CAD build for the part. Positions are in the model's coordinates, mm. A direction names the side the tool comes from. Round coordinates to 2 decimals unless told otherwise and drop trailing zeros. Loops run counter-clockwise (first coordinate to the right, second up) from the corner with the lowest first, then second, coordinate; pieces in that order, holes last.
from build123d import *

# Parameters (mm, degrees)
F0_W      = 153.5
F0_H      = 82
F1_DEPTH  = 2
F2_R      = 7
F2_R_2    = 1.75
F3_DEPTH  = 2.001
F4_SIZE   = 1.99999
F5_R      = 2
F6_DEPTH  = 33
F7_W      = 153.5
F7_H      = 82
F7_W_2    = 149.5
F7_H_2    = 78
F8_DEPTH  = 31
F10_DEPTH = 82.001
F12_DEPTH = 153.501
F13_W     = 56
F13_H     = 56
F13_W_2   = 52
F13_H_2   = 52
F14_DEPTH = 30
F16_DEPTH = 82.001
F17_R     = 5


# Not quite as in the source:
# - a fillet or chamfer is up to 0.001 mm smaller than in the source, because OpenCascade refuses the exact size


with BuildPart() as f1:
    # F0 (on Top) → F1 (new body)
    with BuildSketch(Plane.XY):
        Rectangle(F0_W, F0_H)
    extrude(amount=F1_DEPTH)

    # F2 (on face) → F3 (cut, through all)
    with BuildSketch(Plane.XY.offset(2)):
        with Locations((-48.75, -13)):
            Circle(F2_R)
        with Locations((-68.75, -13)):
            Circle(F2_R_2)
        with Locations((-28.75, -13)):
            Circle(F2_R_2)
    extrude(amount=-F3_DEPTH, mode=Mode.SUBTRACT)

    # F4 (size 2 in the source; OpenCascade refuses exactly that, so slightly less here)
    f4_edges = [f1.edges().sort_by_distance(p)[0] for p in [
        (-70.5, -13, 0),
        (-30.5, -13, 0),
    ]]
    chamfer(f4_edges, length=F4_SIZE)

    # F5 (on face) → F6 (join)
    with BuildSketch(Plane.XY.offset(2)):
        with Locations((-74.75, 39)):
            Circle(F5_R)
        with Locations((74.75, 39)):
            Circle(F5_R)
        with Locations((-74.75, -39)):
            Circle(F5_R)
        with Locations((74.75, -39)):
            Circle(F5_R)
    extrude(amount=F6_DEPTH)

    # F7 (on face) → F8 (join)
    with BuildSketch(Plane.XY.offset(2)):
        Rectangle(F7_W, F7_H)
        Rectangle(F7_W_2, F7_H_2, mode=Mode.SUBTRACT)
    extrude(amount=F8_DEPTH)

    # F9 (on face) → F10 (cut, through all)
    with BuildSketch(Plane.XZ.offset(41)):
        with BuildLine():
            Line((70, 33), (-70, 33))
            ThreePointArc((-70, 33), (0, 5), (70, 33))
        make_face()
    extrude(amount=-F10_DEPTH, mode=Mode.SUBTRACT)

    # F11 (on face) → F12 (cut, through all)
    with BuildSketch(Plane.YZ.offset(76.75)):
        with BuildLine():
            Line((35, 33), (-35, 33))
            ThreePointArc((-35, 33), (0, 5), (35, 33))
        make_face()
    extrude(amount=-F12_DEPTH, mode=Mode.SUBTRACT)

    # F13 (on face) → F14 (join)
    with BuildSketch(Plane.XY.offset(2)):
        with Locations((-48.75, -13)):
            Rectangle(F13_W, F13_H)
        with Locations((-48.75, -13)):
            Rectangle(F13_W_2, F13_H_2, mode=Mode.SUBTRACT)
    extrude(amount=F14_DEPTH)

    # F15 (on face) → F16 (cut, through all)
    with BuildSketch(Plane.XZ.offset(41)):
        Polygon((-20.75, 28), (-20.75, 32), (-44.8423758792, 32), align=None)
    extrude(amount=-F16_DEPTH, mode=Mode.SUBTRACT)

    # F17
    f17_edges = [f1.edges().sort_by_distance(p)[0] for p in [
        (-20.75, -40, 7.143634),
        (-75.75, 15, 8.286419),
    ]]
    fillet(f17_edges, radius=F17_R)


solid = f1.part
Item 1: Mould opens along X. For faces 5 (the cylindrical face through (-75.74, 17.83, 12.85)), 6 (the flat face through (-49, 15, 17)), 7 (the flat face through (76.75, -1, 2)) say: released by +X, released by -X, zero draft, split by the parting line, or undercut.
Verdict:
face 5: zero draft
face 6: undercut
face 7: released by +X
Item 2: Cut at C-C (x = -48.75). List the corners of the cut face in (y, z), plus the area to 3 significant figures.
Verdict:
outline: (-41, 0) - (-20, 0) - (-20, 2) - (-39, 2) - (-39, 32) - (-41, 32) - close; (-6, 0) - (41, 0) - (41, 17.47) - (39, 17.47) - (39, 2) - (15, 2) - (15, 32) - (13, 32) - (13, 2) - (-6, 2) - close
area: 287 mm2
Item 3: Cut at D-D (y = -28.5). List the corners of the cut face in (x, z), plus the area to 3 significant figures.
Verdict:
outline: (-76.75, 0) - (76.75, 0) - (76.75, 19.09) - (74.75, 19.09) - (74.75, 2) - (-20.75, 2) - (-20.75, 28) - (-22.75, 28.33) - (-22.75, 2) - (-74.75, 2) - (-74.75, 32) - (-76.75, 32) - close
area: 454 mm2
Item 4: Wall check: L1, parallel to X at y = -13, z = 2.05; L2, parallel to Y at x = -69, z = 13; L3, parallel to X at y = -29.5, z = 26. Give the ranges that are in metal, low to high.
Verdict:
L1: x = -76.75 to -74.75, -22.75 to -20.75, 74.75 to 76.75
L2: y = -41 to -39, 13 to 15, 39 to 41
L3: x = -76.75 to -74.75, -22.75 to -20.75
Item 5: Flat gauge pins, fed straight in: P1, Ø11, axis at x = -48.75, y = -13, coming from the +Z side; P2, Ø6, axis at x = -34, y = -29, coming from the +Z side; P3, Ø5.5, axis at x = -68.75, y = -13, coming from the -Z side; P4, Ø2, axis at x = -71.5, y = -40, coming from the +Z side. Where does each tip first touch, or does it go through?
Verdict:
P1: passes through
P2: stops at z = 2
P3: stops at z = 1
P4: stops at z = 33
Item 6: Cut at A-A (z = 9). State how many separate pieces and enclosed holes the cut face has, plus the area to 3 significant figures.
Verdict:
separate pieces: 3
enclosed holes: 1
area: 875 mm2
Item 7: 3-axis set-ups, long thin cutter, end or side, ignore diameter. For faces 1 (the flat face through (-22.14, -13.13, 28.23)), 2 (the flat face through (-75, -2, 32)), 3 (the flat face through (75, 39, 35)), 4 (the cylindrical face through (73.532, 37.413, 20.867)): which of +Z, -Z, +X, -X, +Y, -Y reach the whole face in a straight line?
Verdict:
face 1: +Z, +Y, -Y
face 2: +Z, +X, -X
face 3: +Z, +X, -X, +Y, -Y
face 4: +Z
